Autodesk Inventor part; units mm, degrees
ref_plane "工作平面2" through (-13.4156, -13.4156, 7) normal (0, 0, 1) x (1, -0.0000484, 0)
ref_plane "工作平面3" through (0, 0, 7) normal (0, 0, 1) x (1, 0, 0)
ref_plane "工作平面4" through (-7.4754, -7.4754, 19) normal (0, 0, 1) x (1, -0.0000484, 0)
sketch "草圖1" plane through (0, 0, 0) normal (0, 0, 1) x (1, 0, 0)
  circle A0 centre (0, 0) radius 19.6
  circle A1 centre (0, 0) radius 41.5
  dimension "d0" = 39.2
  dimension "d1" = 83
extrude "擠出1" add sketch "草圖1" along normal blind 5
sketch "草圖2" plane through (0, 0, 0) normal (0, 0, -1) x (-1, 0, 0)
  circle A0 centre (0, 0) radius 41.5
extrude "擠出2" add sketch "草圖2" along normal blind 4
sketch "草圖4" plane through (0, 0, 5) normal (0, 0, 1) x (1, 0, 0)
  circle A0 centre (0, 0) radius 41.5
  circle A1 centre (0, 0) radius 37.5
  dimension "d14" = 4
extrude "擠出4" add sketch "草圖4" along normal blind 47.5
sketch "草圖5" plane through (0, 0, 5) normal (0, 0, 1) x (1, 0, 0)
  circle A0 centre (0, 0) radius 37.5
  circle A1 centre (0, 0) radius 33
  dimension "d17" = 4.5
extrude "擠出5" add sketch "草圖5" along normal blind 31.5
sketch "草圖6" plane through (0, 0, -4) normal (0, 0, -1) x (-1, 0, 0)
  line L0 (-66.5, 15.075) -> (-66.5, -15.075)
  line L1 (-66.5, 15.075) -> (-38.6652, 15.075)
  circle A0 centre (0, 0) radius 41.5
  line L2 (-66.5, -15.075) -> (-38.6652, -15.075)
  point P0 (-41.5, 0)
  dimension "d20" = 30.15
  dimension "d22" = 15.075
  dimension "d25" = 25
extrude "擠出6" add sketch "草圖6" against normal up to surface (56.5 mm away) contours L1 A0 L2 L0
sketch "草圖7" plane through (66.5, -15.075, -4) normal (1, 0, 0) x (0, 0, -1)
  line L0 (-56.5, 30.15) -> (-56.5, 0)
  line L1 (0, 0) -> (-56.5, 0)
  line L2 (0, 30.15) -> (0, 0)
  line L3 (0, 30.15) -> (-56.5, 30.15)
  line L4 (-51.5, 5.075) -> (-31.5, 5.075)
  line L5 (-31.5, 5.075) -> (-31.5, 25.075)
  line L6 (-31.5, 25.075) -> (-51.5, 25.075)
  line L7 (-51.5, 25.075) -> (-51.5, 5.075)
  line L8 (-51.5, 5.075) -> (-31.5, 25.075) construction
  line L9 (-31.5, 5.075) -> (-51.5, 25.075) construction
  line L10 (-25, 5.075) -> (-5, 5.075)
  line L11 (-5, 5.075) -> (-5, 25.075)
  line L12 (-5, 25.075) -> (-25, 25.075)
  line L13 (-25, 25.075) -> (-25, 5.075)
  line L14 (-25, 5.075) -> (-5, 25.075) construction
  line L15 (-5, 5.075) -> (-25, 25.075) construction
  point P0 (-4, 15.075)
  point P1 (-41.5, 15.075)
  point P2 (-15, 15.075)
  dimension "d26" = 20
  dimension "d27" = 20
  dimension "d28" = 20
  dimension "d29" = 5
  dimension "d30" = 5.075
  dimension "d31" = 5
  dimension "d85" = 20
extrude "擠出7" cut sketch "草圖7" against normal blind 20 contours L7 L6 L5 L4 | L13 L12 L11 L10
fillet "圓角1" radius 2 7 edges at (52.5826, 15.075, -4) (-41.5, 0, -4) (52.5826, -15.075, -4) (38.6652, 15.075, 24.25) (52.5826, 15.075, 52.5) (-41.5, 0, 52.5) (52.5826, -15.075, 52.5)
sketch "草圖8" plane through (0, 0, 52.5) normal (0, 0, 1) x (1, 0, 0)
  line L0 (52.954, -6.0091) -> (44.994, -6.0078)
  line L1 (52.954, -6.0091) -> (52.955, 0.0909)
  line L2 (44.995, 0.0922) -> (52.955, 0.0909)
  line L3 (44.994, -6.0078) -> (44.995, 0.0922)
  circle A0 centre (48.975, -7.075) radius 1.5
  circle A1 centre (48.975, 7.075) radius 1.5
  line L4 (38.6652, -15.075) -> (66.5, -15.075)
  line L5 (66.5, 15.075) -> (40.0087, 15.075)
  point P0 (0, 0)
  dimension "d36" = 3
  dimension "d37" = 3
  dimension "d38" = 8
  dimension "d39" = 8
extrude "擠出8" cut sketch "草圖8" against normal up to surface (5 mm away) contours A0 L0 | L0 A0 | A1
sketch "草圖9" plane through (38.6652, -15.075, 50.5) normal (0, -1, 0) x (1, 0, 0)
  line L0 (27.8348, -29.5) -> (27.8348, -49.5)
  line L1 (27.8348, -29.5) -> (7.8348, -29.5)
  line L2 (7.8348, -29.5) -> (7.8348, -49.5)
  line L3 (27.8348, -49.5) -> (7.8348, -49.5)
  line L4 (27.8348, -3) -> (27.8348, -23)
  line L5 (27.8348, -3) -> (7.8348, -3)
  line L6 (7.8348, -3) -> (7.8348, -23)
  line L7 (27.8348, -23) -> (7.8348, -23)
  circle A0 centre (17.8294, -39.425) radius 2.1
  circle A1 centre (17.8294, -13.075) radius 2.1
  point P0 (-38.6652, -50.5)
  dimension "d42" = 4.2
  dimension "d43" = 4.2
extrude "擠出9" cut sketch "草圖9" against normal through all contours A0 | A1
sketch "草圖10" plane through (38.6652, -15.075, 50.5) normal (0, -1, 0) x (1, 0, 0)
  circle A0 centre (17.8294, -39.425) radius 2.1
  circle A1 centre (17.8294, -39.425) radius 3.65
  circle A2 centre (17.8294, -13.075) radius 2.1
  circle A3 centre (17.8294, -13.075) radius 3.65
  point P0 (-38.6652, -50.5)
  dimension "d46" = 7.3
  dimension "d47" = 7.3
extrude "擠出10" cut sketch "草圖10" against normal blind 3
mirror "鏡射1" about plane through (0, 0, 0) normal (0, 1, 0) of "擠出10"
sketch "草圖14" plane through (0, 0, 5) normal (0, 0, 1) x (1, 0, 0)
  circle A0 centre (0, 0) radius 19.6
extrude "擠出13" add sketch "草圖14" against normal up to surface (9 mm away)
sketch "草圖15" plane through (0, 0, -4) normal (0, 0, -1) x (-1, 0, 0)
  circle A0 centre (0, 0) radius 13.5
  dimension "d64" = 27
extrude "擠出14" cut sketch "草圖15" against normal up to surface (9 mm away)
sketch "草圖16" plane through (0, 0, 5) normal (0, 0, 1) x (1, 0, 0)
  circle A0 centre (0, 0) radius 18.415
  circle A1 centre (0, 0) radius 13.5
ref_plane "工作平面2" through (-13.4156, -13.4156, 7) normal (0, 0, 1) x (1, -0.0000484, 0)
extrude "擠出15" add sketch "草圖16" along normal up to surface (2 mm away)
ref_plane "工作平面3" through (0, 0, 7) normal (0, 0, 1) x (1, 0, 0)
sketch "草圖17" plane through (0, 0, 7) normal (0, 0, 1) x (1, 0, 0)
  circle A0 centre (0, 0) radius 7.575
  circle A1 centre (0, 0) radius 18.415
  dimension "d71" = 15.15
extrude "擠出16" add sketch "草圖17" along normal blind 3
sketch "草圖18" plane through (0, 0, 10) normal (0, 0, 1) x (1, 0, 0)
  circle A0 centre (0, 0) radius 7.575
  circle A1 centre (0, 0) radius 10.575
  point P0 (0, 0)
  dimension "d74" = 3
ref_plane "工作平面4" through (-7.4754, -7.4754, 19) normal (0, 0, 1) x (1, -0.0000484, 0)
extrude "擠出17" add sketch "草圖18" along normal up to surface (9 mm away)
fillet "圓角3" radius 3 2 edges at (-18.415, 0, 5) (-10.575, 0, 10)
chamfer "倒角1" distance 1 angle 45 1 edges at (13.5, 0, -4)
thread "螺紋1"
thread "螺紋2"
equation "\"d27\" = d26"
equation "\"d28\" = d26"
equation "\"d36\" = d37"
properties part number "j2 arm part_3D 列印"
Can you work these out from the model? Positions are in its coordinate system, mm. A direction names the side the tool comes from. Round coordinates to 2 decimals unless told otherwise and drop trailing zeros. Write each loop counter-clockwise with the first axis right and the second up, starting at its lowest first coordinate (ties: lowest second). Pieces come first, ordered by that corner, then holes. Notation, with made-up numbers: M 33.5,67 L 71.5,67 A5 ccw 71.5,76 Z; hole C 83.25,73.5 d4. An arc over 180 degrees is marked long. Use a Markdown table: item, result.
Item 1: Which directions (+Z, -Z, +X, -X, +Y, -Y) give clear straight access to the entire face, cutting with the end or side of a thin tool? Please do faces 5 (the face through (47.87, -6.06, 50.04)), 6 (the face through (57, 0, 27.5)), 7 (the face through (6, -6, 7)), 8 (the face through (53.8, -13.6, 13.54)).
Found:
| item | result |
|---|---|
| face 5 | +Z |
| face 6 | +X |
| face 7 | -Z |
| face 8 | -Y |
Item 2: We'd pull the mould along X, two halves only. Please class faces 1 (the face through (58.434, 11.023, 10.271)), 2 (the face through (-4.88, -37.18, 44.39)), 3 (the face through (46.5, 0, 38)), 4 (the face through (59, -10, 11)): released by +X, released by -X, zero draft, split by the parting line, or undercut.
Found:
| item | result |
|---|---|
| face 1 | undercut |
| face 2 | undercut |
| face 3 | released by +X |
| face 4 | zero draft |
Item 3: For pin 1 Ø22 at (x, z) = (53.5, 34) entering from +Y (3 decimals); pin 2 Ø1 at (y, z) = (-25, 9.5) entering from -X; pin 3 Ø1 at (y, z) = (4, 7.5) entering from +X; pin 4 Ø13.5 at (x, y) = (0, 0) entering from +Z, each with a flat end and sliding along its axis, tell me the tip position at first contact or that it passes through.
Found:
| item | result |
|---|---|
| pin 1 | stops at y = 15.075 |
| pin 2 | stops at x = -33.5 |
| pin 3 | stops at x = 46.5 |
| pin 4 | passes through |
Item 4: If I drill on line 1 along Y through (x, z) = (10, 6); line 2 along Y through (x, z) = (59, 42) (3 decimals); line 3 along Y through (x, z) = (0, 45.25), over which ranges is the centre line in solid material (lowest first)? Write a range as [from, to].
Found:
| item | result |
|---|---|
| line 1 | y = [-40.28, -31.45], [-16.37, -9.07], [9.07, 16.37], [31.45, 40.28] |
| line 2 | y = [-15.075, -10], [10, 15.075] |
| line 3 | y = [-41.5, -37.5], [37.5, 41.5] |
Item 5: I want a section at A-A (z = 22.5). List the corners of the cut face in (x, y) for me (3 decimals).
Found:
| item | result |
|---|---|
| outline | M 38.169,16.29 A41.5 ccw long 38.665,-15.075 L 66.5,-15.075 L 66.5,15.075 L 40.009,15.075 A2 cw Z; hole C 0,0 d66 |
